Source: three-view drawing plus pictorial views. Frame: mm from the lowest corner of the part. Round coordinates to 2 decimals unless told otherwise and drop trailing zeros. Loops run counter-clockwise (first coordinate to the right, second up) from the corner with the lowest first, then second, coordinate; pieces in that order, holes last. Notation, with made-up numbers: (56.5, -24.5) -> (107.5, -24.5) arc R23 ccw to (107.5, 4.5) -> close; hole circle Ø10 at (67.5, 8.25). An arc over 180 degrees is marked (long way). Answer in a Markdown table with one row per item.
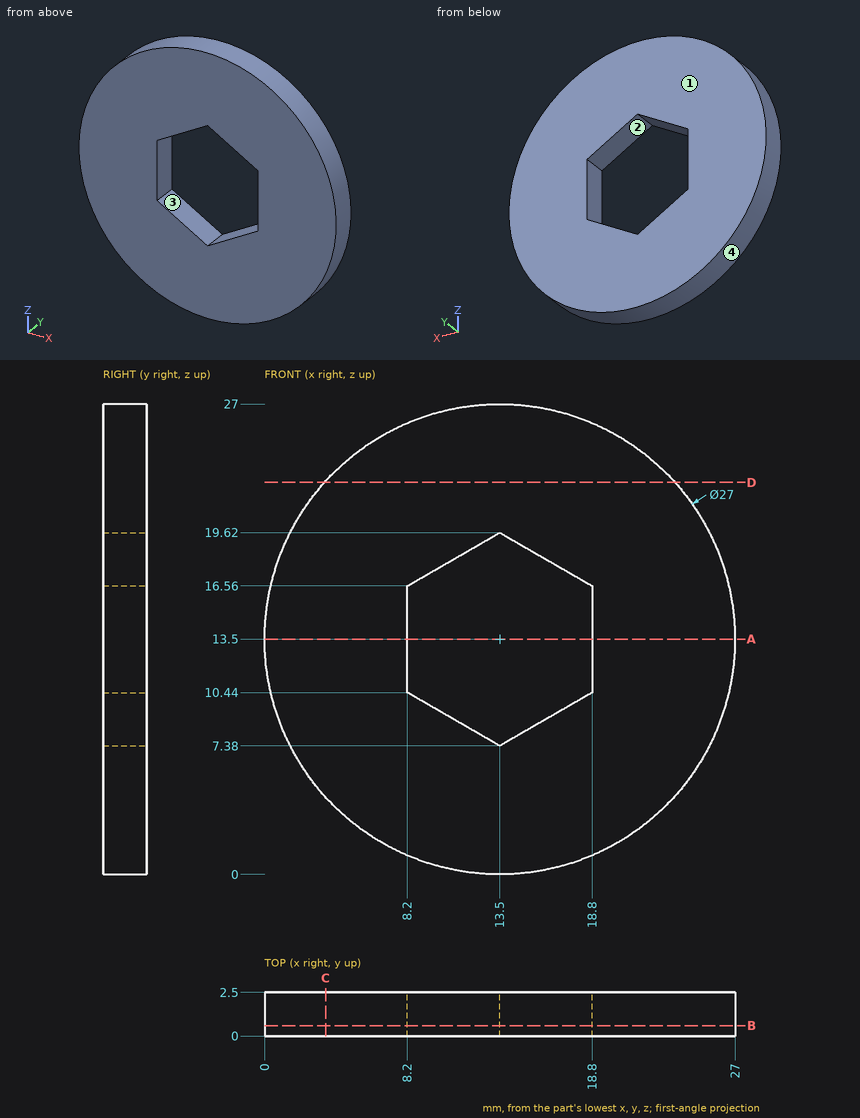
Item 1: Line query: probe 1 along Z at (x, y) = (14.75, 0.5); probe 2 along Z at (x, y) = (8.5, 1.55); probe 3 along X at (y, z) = (1.8, 16.25). Output: solid intervals per line, ascending. Write a range as [from, to].
Answer:
| item | result |
|---|---|
| probe 1 | z = [0.06, 8.1], [18.9, 26.94] |
| probe 2 | z = [0.96, 10.27], [16.73, 26.04] |
| probe 3 | x = [0.28, 8.2], [18.8, 26.72] |
Item 2: Draft query along X for the marked faces 1, 2, 3 and 4. Return one class per face: pulls with the +X half, pulls with the -X half, needs draft (parallel to the pull), parting line crosses it, or undercut.
Answer:
| item | result |
|---|---|
| face 1 | needs draft |
| face 2 | undercut |
| face 3 | undercut |
| face 4 | parting line crosses it |
Item 3: Cut plane B-B (y = 0.6). Output: boundary loops of the cut face in (x, z).
Answer:
| item | result |
|---|---|
| outline | circle Ø27 at (13.5, 13.5); hole (8.2, 10.44) -> (13.5, 7.38) -> (18.8, 10.44) -> (18.8, 16.56) -> (13.5, 19.62) -> (8.2, 16.56) -> close |
Item 4: Cut plane A-A (z = 13.5). Output: boundary loops of the cut face in (x, y).
Answer:
| item | result |
|---|---|
| outline | (0, 0) -> (8.2, 0) -> (8.2, 2.5) -> (0, 2.5) -> close; (18.8, 0) -> (27, 0) -> (27, 2.5) -> (18.8, 2.5) -> close |
Item 5: Cut plane D-D (z = 22.5). Output: boundary loops of the cut face in (x, y).
Answer:
| item | result |
|---|---|
| outline | (3.44, 0) -> (23.56, 0) -> (23.56, 2.5) -> (3.44, 2.5) -> close |
Item 6: Cut plane C-C (x = 3.5). Output: boundary loops of the cut face in (y, z).
Answer:
| item | result |
|---|---|
| outline | (0, 4.43) -> (2.5, 4.43) -> (2.5, 22.57) -> (0, 22.57) -> close |
